Read the model definition and answer for the solid it produces. Units are mm, in the model's axes. Face numbers are marked on the shaded views. A direction names the side the tool comes from. Round coordinates to 2 decimals unless told otherwise and drop trailing zeros. Order: outer loops, then holes, each group sorted by start corner. A loop starts at its lowest first (then second) coordinate and runs counter-clockwise, first axis right, second up. Notation, with made-up numbers: (26.25, -1) - (85.25, -1) arc R25 ccw to (85.25, 31) - close; hole circle Ø8 at (21.25, 63). An arc over 180 degrees is marked (long way). One line per question, with ' | ' between items. Start each with the question number.
1) The part is cut by section B-B, the plane x = 67.5. Give the vertices of the cut face in (y, z).
2) Straight lines are drawn through the part: line 1 (X direction, y = -30, z = 25); line 2 (Y direction, x = -67.5, z = 32.5); line 3 (Y direction, x = 12, z = 46.5). For each, find the intervals that lie inside material, in ascending order. Write a range as from..to.
3) A flat-ended cylindrical pin translates along its axis: pin 1 (1 mm diameter, centred on x = 89, y = -22, fed in from +Z). Find the tip coordinate at first contact, or state that the pin passes through.
4) The part is cut by section A-A, the plane y = -17. Give the vertices of the cut face in (x, z).
5) The mould has two halves that part along Y. Classify the marked faces 3, 4 and 5: pulls with the +Y half, pulls with the -Y half, needs draft (parallel to the pull), parting line crosses it, or undercut.
6) For the marked faces 1 and 2, determine the directions among +Z, -Z, +X, -X, +Y, -Y from which every point of the face is accessible in a straight line to the end or side of a thin tool.
7) The part is cut by section C-C, the plane z = 11.5. Give the vertices of the cut face in (x, y).
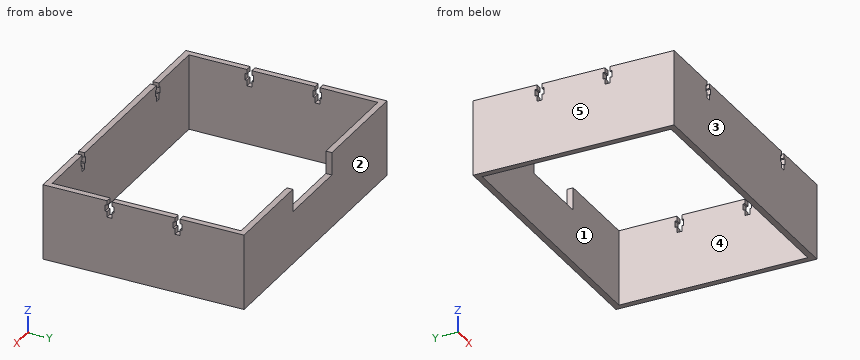
from build123d import *

# Parameters (mm, degrees)
ESQUISSE2_W             = 183
ESQUISSE2_H             = 133
BOSS_EXTRU_2_DEPTH      = 50
ESQUISSE3_W             = 50
ESQUISSE3_H             = 15
ENL_V_MAT_EXTRU_1_DEPTH = 50
ENL_V_MAT_EXTRU_3_DEPTH = 4
ENL_V_MAT_EXTRU_4_DEPTH = 4
ENL_V_MAT_EXTRU_5_DEPTH = 4


with BuildPart() as part:
    # Esquisse2 → Boss.-Extru.2 (new body)
    with BuildSketch(Plane.XY):
        Rectangle(ESQUISSE2_W, ESQUISSE2_H)
        Polygon((-85.996240602, -62.5), (-87.5, -62.5), (-87.5, 62.5), (87.5, 62.5), (87.5, -62.5), align=None, mode=Mode.SUBTRACT)
    extrude(amount=BOSS_EXTRU_2_DEPTH)

    # Esquisse3 → Enlèv. mat.-Extru.1 (cut)
    with BuildSketch(Plane(origin=(0, 66.5, 0), x_dir=(1, 0, 0), z_dir=(0, 1, 0))):
        with Locations((4, -42.5)):
            Rectangle(ESQUISSE3_W, ESQUISSE3_H)
    extrude(amount=-ENL_V_MAT_EXTRU_1_DEPTH, mode=Mode.SUBTRACT)

    # Esquisse6 → Enlèv. mat.-Extru.3 (cut)
    with BuildSketch(Plane(origin=(91.5, 0, 0), x_dir=(0, 0, -1), z_dir=(1, 0, 0))):
        Polygon((-50, 20.9), (-47, 20.9), (-47, 19.65), (-42.8, 19.65), (-42.8, 20.9), (-39, 20.9), (-39, 24.1), (-42.8, 24.1), (-42.8, 25.35), (-47, 25.35), (-47, 24.1), (-50, 24.1), align=None)
        Polygon((-50, -24.1), (-47, -24.1), (-47, -25.35), (-42.8, -25.35), (-42.8, -24.1), (-39, -24.1), (-39, -20.9), (-42.8, -20.9), (-42.8, -19.65), (-47, -19.65), (-47, -20.9), (-50, -20.9), align=None)
    extrude(amount=-ENL_V_MAT_EXTRU_3_DEPTH, mode=Mode.SUBTRACT)

    # Esquisse7 → Enlèv. mat.-Extru.4 (cut)
    with BuildSketch(Plane.ZY.offset(91.5)):
        Polygon((47, 20.9), (50, 20.9), (50, 24.1), (47, 24.1), (47, 25.35), (42.8, 25.35), (42.8, 24.1), (39, 24.1), (39, 20.9), (42.8, 20.9), (42.8, 19.65), (47, 19.65), align=None)
        Polygon((47, -24.1), (50, -24.1), (50, -20.9), (47, -20.9), (47, -19.65), (42.8, -19.65), (42.8, -20.9), (39, -20.9), (39, -24.1), (42.8, -24.1), (42.8, -25.35), (47, -25.35), align=None)
    extrude(amount=-ENL_V_MAT_EXTRU_4_DEPTH, mode=Mode.SUBTRACT)

    # Esquisse9 → Enlèv. mat.-Extru.5 (cut)
    with BuildSketch(Plane.XZ.offset(66.5)):
        Polygon((-49.1, 50), (-45.9, 50), (-45.9, 47), (-44.65, 47), (-44.65, 42.8), (-45.9, 42.8), (-45.9, 39), (-49.1, 39), (-49.1, 42.8), (-50.35, 42.8), (-50.35, 47), (-49.1, 47), align=None)
        Polygon((45.9, 50), (45.9, 47), (44.65, 47), (44.65, 42.8), (45.9, 42.8), (45.9, 39), (49.1, 39), (49.1, 42.8), (50.35, 42.8), (50.35, 47), (49.1, 47), (49.1, 50), align=None)
    extrude(amount=-ENL_V_MAT_EXTRU_5_DEPTH, mode=Mode.SUBTRACT)


solid = part.part
Values:
1) outline: (-66.5, 0) - (-62.5, 0) - (-62.5, 50) - (-66.5, 50) - close; (62.5, 0) - (66.5, 0) - (66.5, 50) - (62.5, 50) - close
2) line 1: x = -91.5..-87.5, 87.5..91.5 | line 2: y = -66.5..-62.5, 62.5..66.5 | line 3: y = -66.5..-62.5
3) pin 1: stops at z = 39
4) outline: (-91.5, 0) - (-87.5, 0) - (-87.5, 50) - (-91.5, 50) - close; (87.5, 0) - (91.5, 0) - (91.5, 50) - (87.5, 50) - close
5) face 3: pulls with the -Y half | face 4: undercut | face 5: needs draft
6) face 1: +Z, -Z | face 2: +Z, -Z, +X, -X, +Y
7) outline: (-91.5, -66.5) - (91.5, -66.5) - (91.5, 66.5) - (-91.5, 66.5) - close; hole (-87.5, -62.5) - (87.5, -62.5) - (87.5, 62.5) - (-87.5, 62.5) - close
